```python
from build123d import *

# Parameters (mm, degrees)
CHAFL_N1_SIZE = 0.396875


with BuildPart() as part:
    # Croquis1 → Revolución1 (revolve)
    with BuildSketch(Plane(origin=(0, 0, 0), x_dir=(0, 0, -1), z_dir=(1, 0, 0)), mode=Mode.PRIVATE) as revoluci_n1_sk:
        with BuildLine():
            Line((-15.24, 0), (-15.24, 3.175))
            Line((-15.24, 3.175), (3.81, 3.175))
            ThreePointArc((3.81, 3.175), (4.650083071, 2.302185344), (5.818206951, 1.9812))
            Line((5.818206951, 1.9812), (15.24, 1.9812))
            Line((15.24, 1.9812), (15.24, 0))
            Line((15.24, 0), (-15.24, 0))
        make_face()
    revolve(revoluci_n1_sk.sketch.rotate(Axis((0, 0, -127), (0, 0, 1)), 90), axis=Axis((0, 0, -127), (0, 0, 1)))

    # Croquis4 → Cortar-Revolución1 (revolve, cut)
    with BuildSketch(Plane(origin=(0, 0, 0), x_dir=(0, 0, -1), z_dir=(1, 0, 0)), mode=Mode.PRIVATE) as cortar_revoluci_n1_sk:
        with BuildLine():
            ThreePointArc((15.24, 1.722711816), (14.861646983, 0.898025612), (14.732, 0))
            Line((14.732, 0), (15.24, 0))
            Line((15.24, 0), (15.24, 1.722711816))
        make_face()
        with BuildLine():
            ThreePointArc((14.732, 0), (14.861646983, 0.898025612), (15.24, 1.722711816))
            Line((15.24, 1.722711816), (15.24, 0))
            Line((15.24, 0), (14.732, 0))
        make_face()
    revolve(cortar_revoluci_n1_sk.sketch.rotate(Axis((0, 0, -15.24), (0, 0, 1)), 180), axis=Axis((0, 0, -15.24), (0, 0, 1)), mode=Mode.SUBTRACT)

    # Chaflán1
    chafl_n1_edges = [part.edges().sort_by_distance(p)[0] for p in [
        (3.175, 0, 15.24),
    ]]
    chamfer(chafl_n1_edges, length=CHAFL_N1_SIZE)


solid = part.part
```
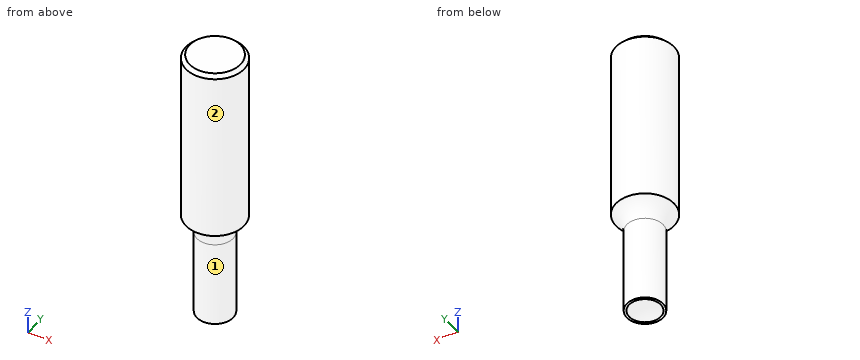
The model under review builds one solid part; all positions refer to its coordinate system, in mm. Face numbers are marked on the shaded views. A direction names the side the tool comes from. Coordinates: 2 decimals unless noted, no trailing zeros. Write each loop counter-clockwise with the first axis right and the second up, starting at its lowest first coordinate (ties: lowest second). Pieces come first, ordered by that corner, then holes.
1) Machinability: for the marked faces 1 and 2, which of the approach directions +Z, -Z, +X, -X, +Y, -Y give a long, thin tool a straight path to every point of the face, cutting with its end or side? Answer none if there is none.
2) We need section A-A on y = 0. State the section outline as (x, z) points (3 decimals), then the cut area to 3 significant figures.
3) To check wall thickness, follow probe 1 along X at (y, z) = (-1.25, 13); probe 2 along Z at (x, y) = (1.5, -2); probe 3 along Z at (x, y) = (-0.5, 1). State the ranges of each line that lie inside material, in increasing order.
4) We need section C-C on z = -3. State the section outline as (x, y) points (3 decimals), then the cut area to 3 significant figures.
Answer list:
1. face 1: -Z
1. face 2: +Z, -Z
2. outline: (-3.175, -3.81) arc R2.286 cw to (-1.981, -5.818) - (-1.981, -15.24) - (-1.723, -15.24) arc R3.175 cw to (1.723, -15.24) - (1.981, -15.24) - (1.981, -5.818) arc R2.286 cw to (3.175, -3.81) - (3.175, 14.843) - (2.778, 15.24) - (-2.778, 15.24) - (-3.175, 14.843) - close
2. area: 166 mm2
3. probe 1: x = -2.92 to 2.92
3. probe 2: z = -4.37 to 15.24
3. probe 3: z = -14.94 to 15.24
4. outline: circle Ø6.35 at (0, 0)
4. area: 31.7 mm2
